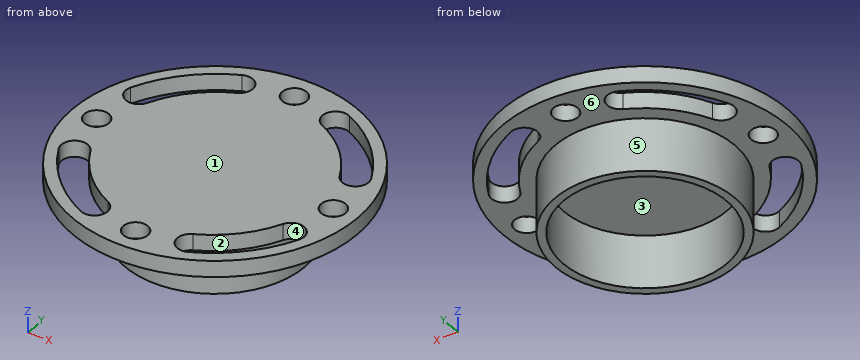
from build123d import *

# Parameters (mm, degrees)
SKETCH_1_R          = 22.1
SKETCH_1_R_2        = 20.1
EXTRUDE_1_DEPTH     = 13
SKETCH_3_R          = 35
EXTRUDE_2_DEPTH     = 4
CUT_EXTRUDE_2_DEPTH = 4
SKETCH_7_R          = 2.5
CUT_EXTRUDE_3_DEPTH = 4
SKETCH_8_R          = 3
CUT_EXTRUDE_4_DEPTH = 4


with BuildPart() as part:
    # 草图1 → 凸台-拉伸1 (new body)
    with BuildSketch(Plane.XY):
        Circle(SKETCH_1_R)
        Circle(SKETCH_1_R_2, mode=Mode.SUBTRACT)
    extrude(amount=-EXTRUDE_1_DEPTH)

    # 草图3 → 凸台-拉伸2 (add)
    with BuildSketch(Plane.XY):
        Circle(SKETCH_3_R)
    extrude(amount=EXTRUDE_2_DEPTH)

    # 草图6 → 切除-拉伸2 (cut)
    with BuildSketch(Plane.XY):
        with BuildLine():
            ThreePointArc((-13.13288474, 29.454672407), (-22.761081404, 22.761081404), (-29.454672407, 13.13288474))
            ThreePointArc((-29.454672407, 13.13288474), (-27.853665751, 8.824546582), (-23.545327593, 10.425553238))
            ThreePointArc((-23.545327593, 10.425553238), (-18.164887326, 18.164887326), (-10.425553238, 23.545327593))
            ThreePointArc((-10.425553238, 23.545327593), (-8.824546582, 27.853665751), (-13.13288474, 29.454672407))
        make_face()
        with BuildLine():
            ThreePointArc((29.448536872, 13.146197524), (22.743952769, 22.743952769), (13.146197524, 29.448536872))
            ThreePointArc((13.146197524, 29.448536872), (8.830682117, 27.866978535), (10.412240454, 23.551463128))
            ThreePointArc((10.412240454, 23.551463128), (18.147758691, 18.147758691), (23.551463128, 10.412240454))
            ThreePointArc((23.551463128, 10.412240454), (27.866978535, 8.830682117), (29.448536872, 13.146197524))
        make_face()
        with BuildLine():
            ThreePointArc((13.174546029, -29.435227837), (22.707404076, -22.707404076), (29.435227837, -13.174546029))
            ThreePointArc((29.435227837, -13.174546029), (27.895327039, -8.843991153), (23.564772163, -10.38389195))
            ThreePointArc((23.564772163, -10.38389195), (18.111209998, -18.111209998), (10.38389195, -23.564772163))
            ThreePointArc((10.38389195, -23.564772163), (8.843991153, -27.895327039), (13.174546029, -29.435227837))
        make_face()
        with BuildLine():
            ThreePointArc((-29.428635355, -13.188330396), (-22.68959412, -22.68959412), (-13.188330396, -29.428635355))
            ThreePointArc((-13.188330396, -29.428635355), (-8.850583634, -27.909111407), (-10.370107582, -23.571364645))
            ThreePointArc((-10.370107582, -23.571364645), (-18.093400043, -18.093400043), (-23.571364645, -10.370107582))
            ThreePointArc((-23.571364645, -10.370107582), (-27.909111407, -8.850583634), (-29.428635355, -13.188330396))
        make_face()
    extrude(amount=CUT_EXTRUDE_2_DEPTH, mode=Mode.SUBTRACT)

    # 草图7 → 切除-拉伸3 (cut)
    with BuildSketch(Plane(origin=(0, 0, 0), x_dir=(-1, 0, 0), z_dir=(0, 0, -1))):
        with Locations((0, 29)):
            Circle(SKETCH_7_R)
        with Locations((29, 0)):
            Circle(SKETCH_7_R)
        with Locations((0, -29)):
            Circle(SKETCH_7_R)
        with Locations((-29, 0)):
            Circle(SKETCH_7_R)
    extrude(amount=-CUT_EXTRUDE_3_DEPTH, mode=Mode.SUBTRACT)

    # 草图8 → 切除-拉伸4 (cut)
    with BuildSketch(Plane.XY):
        with Locations((0, 29)):
            Circle(SKETCH_8_R)
        with Locations((-29, 0)):
            Circle(SKETCH_8_R)
        with Locations((0, -29)):
            Circle(SKETCH_8_R)
        with Locations((29, 0)):
            Circle(SKETCH_8_R)
    extrude(amount=CUT_EXTRUDE_4_DEPTH, mode=Mode.SUBTRACT)


solid = part.part
Can you work these out from the model? Positions are in its coordinate system, mm. Face numbers are marked on the shaded views. A direction names the side the tool comes from. Coordinates: 2 decimals unless noted, no trailing zeros. Loops run counter-clockwise (first coordinate to the right, second up) from the corner with the lowest first, then second, coordinate; pieces in that order, holes last. Notation, with made-up numbers: (-32.5, 21.5) - (-23.5, 21.5) arc R20 cw to (-23.5, 34.5) - close; hole circle Ø3 at (-40, 36.5). An arc over 180 degrees is marked (long way). Put each result on its own line as item: value. Start each with the question number.
Item 1: Suppose I cut it at B-B (x = -1.5). Please give me the cut outline in (y, z), and give its area (3 significant figures).
Item 2: Suppose I cut it at D-D (z = -6.25). Please give me the cut outline in (x, y).
Item 3: Suppose I cut it at C-C (x = 28). Please give me the cut outline in (y, z).
Item 4: Suppose I cut it at A-A (y = -14.5). Please give me the cut outline in (x, z).
Item 5: If I drill on line 1 along Y through (x, z) = (0, 2.25); line 2 along X through (y, z) = (-11.5, 0.75); line 3 along Y through (x, z) = (20, 3), over which ranges is the centre line in solid material (lowest first)?
Item 6: For pin 1 (5 mm diameter, centred on x = 12.5, y = 27.5, fed in from -Z); pin 2 (4 mm diameter, centred on x = 21, z = -2.5, fed in from +Y), each with a flat end and sliding along its axis, tell me the tip position at first contact or that it passes through.
Item 7: Which directions (+Z, -Z, +X, -X, +Y, -Y) give clear straight access to the entire face, cutting with the end or side of a thin tool? Please do the marked faces 1, 2 and 3.
Item 8: If we mould it in two halves opening along X, with no side actions, what happens to the marked faces 4, 5 and 6? For each: +X half, -X half, draft (parallel to the pull), parting line (faces both ways), or undercut.
Here are the results:
1. outline: (-34.97, 0) - (-31.6, 0) - (-31.6, 4) - (-34.97, 4) - close; (-26.4, 0) - (-22.05, 0) - (-22.05, -13) - (-20.04, -13) - (-20.04, 0) - (20.04, 0) - (20.04, -13) - (22.05, -13) - (22.05, 0) - (26.4, 0) - (26.4, 4) - (-26.4, 4) - close; (31.6, 0) - (34.97, 0) - (34.97, 4) - (31.6, 4) - close
1. area: 290 mm²
2. outline: circle Ø44.2 at (0, 0); hole circle Ø40.2 at (0, 0)
3. outline: (-21, 0) - (-15.88, 0) - (-15.88, 4) - (-21, 4) - close; (-8.9, 0) - (-2.83, 0) - (-2.83, 4) - (-8.9, 4) - close; (2.83, 0) - (8.9, 0) - (8.9, 4) - (2.83, 4) - close; (15.92, 0) - (21, 0) - (21, 4) - (15.92, 4) - close
4. outline: (-31.86, 0) - (-28.76, 0) - (-28.76, 4) - (-31.86, 4) - close; (-21.13, 0) - (-16.68, 0) - (-16.68, -13) - (-13.92, -13) - (-13.92, 0) - (13.92, 0) - (13.92, -13) - (16.68, -13) - (16.68, 0) - (21.16, 0) - (21.16, 4) - (-21.13, 4) - close; (28.77, 0) - (31.86, 0) - (31.86, 4) - (28.77, 4) - close
5. line 1: -35 to -32, -26 to 26, 32 to 35
5. line 2: -33.06 to -29.74, -23 to 23, 29.74 to 33.06
5. line 3: -28.72 to -25.14, -16.02 to 16.1, 25.2 to 28.72
6. pin 1: z = 0
6. pin 2: y = 11.29
7. face 1: +Z, +X, -X, +Y, -Y
7. face 2: +Z, -Z
7. face 3: -Z
8. face 4: undercut
8. face 5: parting line
8. face 6: draft
